from build123d import *

# Parameters (mm, degrees)
SKETCH1_R           = 42.75
BOSS_EXTRUDE1_DEPTH = 5
SKETCH2_R           = 2.8
CUT_EXTRUDE1_DEPTH  = 61.664033826
SKETCH3_R           = 17.5
BOSS_EXTRUDE2_DEPTH = 5
SKETCH4_R           = 19.5
BOSS_EXTRUDE3_DEPTH = 1


with BuildPart() as part:
    # Sketch1 → Boss-Extrude1 (new body)
    with BuildSketch(Plane(origin=(0, 0, 0), x_dir=(1, 0, 0), z_dir=(0, 1, 0))):
        with Locations(Location((0, 0, 0), (0, 0, 270))):
            Circle(SKETCH1_R)
    extrude(amount=BOSS_EXTRUDE1_DEPTH)

    # Sketch2 → Cut-Extrude1 (cut, through all)
    with BuildSketch(Plane(origin=(0, 5, 0), x_dir=(1, 0, 0), z_dir=(0, 1, 0))):
        with Locations(Location((0, 34, 0), (0, 0, 270))):
            Circle(SKETCH2_R)
        with Locations(Location((24.04163056, 24.04163056, 0), (0, 0, 270))):
            Circle(SKETCH2_R)
        with Locations(Location((34, 0, 0), (0, 0, 270))):
            Circle(SKETCH2_R)
        with Locations(Location((24.04163056, -24.04163056, 0), (0, 0, 270))):
            Circle(SKETCH2_R)
        with Locations(Location((0, -34, 0), (0, 0, 270))):
            Circle(SKETCH2_R)
        with Locations(Location((-24.04163056, -24.04163056, 0), (0, 0, 270))):
            Circle(SKETCH2_R)
        with Locations(Location((-34, 0, 0), (0, 0, 270))):
            Circle(SKETCH2_R)
        with Locations(Location((-24.04163056, 24.04163056, 0), (0, 0, 270))):
            Circle(SKETCH2_R)
    extrude(amount=-CUT_EXTRUDE1_DEPTH, mode=Mode.SUBTRACT)

    # Sketch3 → Boss-Extrude2 (add)
    with BuildSketch(Plane(origin=(0, 5, 0), x_dir=(1, 0, 0), z_dir=(0, 1, 0))):
        with Locations(Location((0, 0, 0), (0, 0, 270))):
            Circle(SKETCH3_R)
    extrude(amount=BOSS_EXTRUDE2_DEPTH)

    # Sketch4 → Boss-Extrude3 (add)
    with BuildSketch(Plane(origin=(0, 5, 0), x_dir=(1, 0, 0), z_dir=(0, 1, 0))):
        with Locations(Location((0, 0, 0), (0, 0, 270))):
            Circle(SKETCH4_R)
    extrude(amount=BOSS_EXTRUDE3_DEPTH)


solid = part.part
Work out the finished part from the listing and answer in its coordinate system (mm). A direction names the side the tool comes from. Give positions to 0.01 mm unless a question says otherwise; leave off trailing zeros. Order: outer loops, then holes, each group sorted by start corner. A loop starts at its lowest first (then second) coordinate and runs counter-clockwise, first axis right, second up. Notation, with made-up numbers: (25.5, 21.5) -> (34.5, 21.5) arc R21 cw to (34.5, 41.5) -> close; hole circle Ø4 at (-4, -8.5). An arc over 180 degrees is marked (long way). One line per item, written item: value.
Item 1: Find section D-D, the plane z = 34. Give the vertices of the cut face in (x, y), plus the area to 3 significant figures.
Answer sheet:
outline: (-25.91, 0) -> (-2.8, 0) -> (-2.8, 5) -> (-25.91, 5) -> close; (2.8, 0) -> (25.91, 0) -> (25.91, 5) -> (2.8, 5) -> close
area: 231 mm²
Item 2: Find section A-A, the plane z = 0. Give the vertices of the cut face in (x, y), plus the area to 4 significant figures.
Answer sheet:
outline: (-42.75, 0) -> (-36.8, 0) -> (-36.8, 5) -> (-42.75, 5) -> close; (-31.2, 0) -> (31.2, 0) -> (31.2, 5) -> (19.5, 5) -> (19.5, 6) -> (17.5, 6) -> (17.5, 10) -> (-17.5, 10) -> (-17.5, 6) -> (-19.5, 6) -> (-19.5, 5) -> (-31.2, 5) -> close; (36.8, 0) -> (42.75, 0) -> (42.75, 5) -> (36.8, 5) -> close
area: 550.5 mm²
Item 3: Find section B-B, the plane x = 23. Give the vertices of the cut face in (y, z).
Answer sheet:
outline: (0, -36.04) -> (5, -36.04) -> (5, -26.64) -> (0, -26.64) -> close; (0, -21.44) -> (5, -21.44) -> (5, 21.44) -> (0, 21.44) -> close; (0, 26.64) -> (5, 26.64) -> (5, 36.04) -> (0, 36.04) -> close
Item 4: Straight lines are drawn through the part: probe 1 along X at (y, z) = (2.7, 0); probe 2 along Y at (x, z) = (-27, -8); probe 3 along X at (y, z) = (3.5, 34). For each, find the intervals that lie inside material, in ascending order.
Answer sheet:
probe 1: -42.75 to -36.8, -31.2 to 31.2, 36.8 to 42.75
probe 2: 0 to 5
probe 3: -25.91 to -2.8, 2.8 to 25.91
Item 5: Find section C-C, the plane y = 3.25. State how many separate pieces and enclosed holes the cut face has, plus the area to 3 significant figures.
Answer sheet:
separate pieces: 1
enclosed holes: 8
area: 5,540 mm²
Item 6: Flat-ended cylindrical pins translate along their axes: P1, Ø7.5, axis at x = 0, z = 34, coming from the +Y side; P2, Ø6, axis at x = -30.5, z = 32, coming from the -Y side; P3, Ø3, axis at x = -33.5, y = 2.5, coming from the -Z side; P4, Ø5, axis at x = 24.04, z = 24.04, coming from the -Y side. Find the tip coordinate at first contact, or state that the pin passes through.
Answer sheet:
P1: y = 5
P2: y = 0
P3: z = -28.35
P4: through
Item 7: A tool of negligible diameter and unlimited length cuts with its end or side. For faces 4 (the cylindrical face through (19.334, 5.493, -2.539)), 5 (the cylindrical face through (35.892, 2.535, -2.064)), from which of +Z, -Z, +X, -X, +Y, -Y can it reach the whole face along a straight path? Write none if from no direction.
Answer sheet:
face 4: +Y
face 5: +Y, -Y
Item 8: Determine the mould class of faces 1 (the cylindrical face through (42.386, 2.465, -5.565)), 2 (the flat face through (12, 6, -13)), 3 (the cylindrical face through (22.97, 2.54, 26.63)) for opening direction X: released by +X, released by -X, zero draft, split by the parting line, or undercut.
Answer sheet:
face 1: split by the parting line
face 2: zero draft
face 3: undercut
